The listing builds one solid part. Answer for the finished solid, in the listing's coordinates (mm). Coordinates: 2 decimals unless noted, no trailing zeros. Order: outer loops, then holes, each group sorted by start corner. A loop starts at its lowest first (then second) coordinate and runs counter-clockwise, first axis right, second up.
from build123d import *

# Parameters (mm, degrees)
F1_DEPTH  = 1
F4_DEPTH  = 8
F5_R      = 0.5
F6_W      = 2
F6_H      = 0.5
F7_DEPTH  = 0.5
F8_R      = 0.24999
F9_W      = 2
F9_H      = 3
F10_DEPTH = 2


# Not quite as in the source:
# - a fillet or chamfer is up to 0.001 mm smaller than in the source, because OpenCascade refuses the exact size


with BuildPart() as f1:
    # F0 (on Front) → F1 (new body)
    with BuildSketch(Plane.XZ):
        with BuildLine():
            Line((-42.178902775, 4), (-42.178902775, 0))
            Line((-42.178902775, 0), (-42.178902775, -4))
            Line((-42.178902775, -4), (-39.678902775, -6))
            Line((-39.678902775, -6), (15.821097225, -6))
            Line((15.821097225, -6), (15.821097225, -4.5))
            ThreePointArc((15.821097225, -4.5), (15.9675438344, -4.1464466094), (16.321097225, -4))
            Line((16.321097225, -4), (25.821097225, -4))
            Line((25.821097225, -4), (25.821097225, 0))
            Line((25.821097225, 0), (25.821097225, 4))
            Line((25.821097225, 4), (16.321097225, 4))
            ThreePointArc((16.321097225, 4), (15.9675438344, 4.1464466094), (15.821097225, 4.5))
            Line((15.821097225, 4.5), (15.821097225, 6))
            Line((15.821097225, 6), (-39.678902775, 6))
            Line((-39.678902775, 6), (-42.178902775, 4))
        make_face()
    extrude(amount=F1_DEPTH)



with BuildPart() as f4:
    # F3 (on offset) → F4 (new body)
    with BuildSketch(Plane.YZ.offset(16.5)):
        with BuildLine():
            Line((-1, -6), (3, -6))
            ThreePointArc((3, -6), (4.4142135624, -5.4142135624), (5, -4))
            Line((5, -4), (5, 4))
            ThreePointArc((5, 4), (4.4142135624, 5.4142135624), (3, 6))
            Line((3, 6), (-1, 6))
            ThreePointArc((-1, 6), (-2.4142135624, 5.4142135624), (-3, 4))
            Line((-3, 4), (-3, -4))
            ThreePointArc((-3, -4), (-2.4142135624, -5.4142135624), (-1, -6))
        make_face()
        with BuildLine():
            ThreePointArc((3.5, -3.5), (3.2071067812, -4.2071067812), (2.5, -4.5))
            Line((2.5, -4.5), (-0.5, -4.5))
            ThreePointArc((-0.5, -4.5), (-1.2071067812, -4.2071067812), (-1.5, -3.5))
            Line((-1.5, -3.5), (-1.5, 3.5))
            ThreePointArc((-1.5, 3.5), (-1.2071067812, 4.2071067812), (-0.5, 4.5))
            Line((-0.5, 4.5), (2.5, 4.5))
            ThreePointArc((2.5, 4.5), (3.2071067812, 4.2071067812), (3.5, 3.5))
            Line((3.5, 3.5), (3.5, -3.5))
        make_face(mode=Mode.SUBTRACT)
    extrude(amount=F4_DEPTH)

    # F5
    f5_edges = [f4.edges().sort_by_distance(p)[0] for p in [
        (24.5, -2.414214, 5.414214),
        (24.5, -1.207107, 4.207107),
        (16.5, -1.207107, 4.207107),
        (16.5, -2.414214, 5.414214),
    ]]
    fillet(f5_edges, radius=F5_R)


with BuildPart() as f1_1:
    add(f1.part)

    add(f4.part)  # F7 merges F4
    # F6 (on offset) → F7 (join)
    with BuildSketch(Plane.YZ.offset(16.5)):
        with Locations((-1.159823034, 0)):
            Rectangle(F6_W, F6_H)
    extrude(amount=F7_DEPTH)

    # F8 (radius 0.25 in the source; OpenCascade refuses exactly that, so slightly less here)
    f8_edges = [f1_1.edges().sort_by_distance(p)[0] for p in [
        (17, -1.25, 0.25),
        (17, -1.25, -0.25),
        (16.5, -1.5, -0.25),
        (16.5, -1.5, 0.25),
    ]]
    fillet(f8_edges, radius=F8_R)

    # F9 (on Front) → F10 (join)
    with BuildSketch(Plane.XZ):
        with Locations((-4.178902775, -2)):
            Rectangle(F9_W, F9_H)
    extrude(amount=F10_DEPTH)


solid = f1_1.part
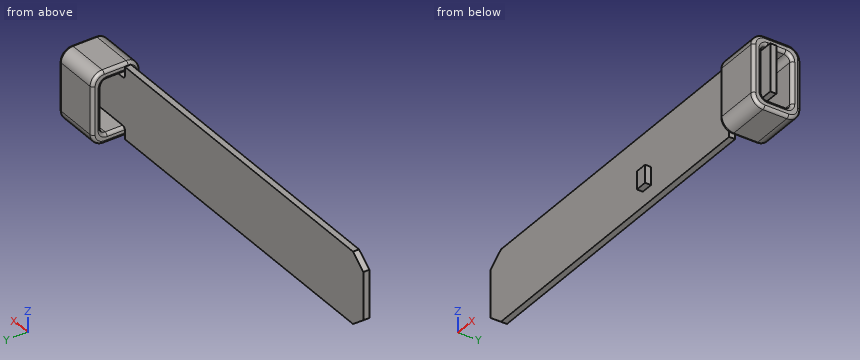
1) Section C-C (x = -33.5) is taken. Give the vertices of the cut face in (y, z).
2) Each of these flat-tipped pins is pushed along its axis until it touches: P1, Ø1, axis at y = -2, z = -0.5, coming from the -X side; P2, Ø0.8, axis at x = -4, y = -1.5, coming from the -Z side; P3, Ø6, axis at x = -13, z = -2, coming from the -Y side. Where does it stop, or does it pass through?
3) Consider L1, parallel to Z at x = -4, y = -1.75; L2, parallel to Y at x = -24, z = 5.25; L3, parallel to X at y = 3.25, z = -5. Determine where each line is inside the solid, lowest interval first.
4) Section B-B (y = 1.5) is taken. Give the vertices of the cut face in (x, z).
5) Section A-A (z = 1.5) is taken. Give the vertices of the cut face in (x, y), then the cut area to 3 significant figures.
Filled sheet:
1. outline: (-1, -6) - (0, -6) - (0, 6) - (-1, 6) - close
2. P1: stops at x = -5.18
2. P2: stops at z = -3.5
2. P3: stops at y = -1
3. L1: z = -3.5 to -0.5
3. L2: y = -1 to 0
3. L3: x = 16.5 to 24.5
4. outline: (16.5, -5.5) arc R0.5 ccw to (17, -6) - (24, -6) arc R0.5 ccw to (24.5, -5.5) - (24.5, -5) arc R0.5 ccw to (24, -4.5) - (17, -4.5) arc R0.5 ccw to (16.5, -5) - close; (16.5, 5) arc R0.5 ccw to (17, 4.5) - (24, 4.5) arc R0.5 ccw to (24.5, 5) - (24.5, 5.5) arc R0.5 ccw to (24, 6) - (17, 6) arc R0.5 ccw to (16.5, 5.5) - close
5. outline: (-42.18, -1) - (25.82, -1) - (25.82, 0) - (-42.18, 0) - close; (16.5, -2.5) arc R0.5 ccw to (17, -3) - (24, -3) arc R0.5 ccw to (24.5, -2.5) - (24.5, -2) arc R0.5 ccw to (24, -1.5) - (17, -1.5) arc R0.5 ccw to (16.5, -2) - close; (16.5, 4) arc R0.5 ccw to (17, 3.5) - (24, 3.5) arc R0.5 ccw to (24.5, 4) - (24.5, 4.5) arc R0.5 ccw to (24, 5) - (17, 5) arc R0.5 ccw to (16.5, 4.5) - close
5. area: 91.6 mm2
